Work out the finished part from the listing and answer in its coordinate system (mm). A direction names the side the tool comes from. Coordinates: 2 decimals unless noted, no trailing zeros. Order: outer loops, then holes, each group sorted by start corner. A loop starts at its lowest first (then second) coordinate and runs counter-clockwise, first axis right, second up. Notation, with made-up numbers: M 17.25,63.5 L 62.25,63.5 A18 cw 62.25,72.5 Z; hole C -40,-20.75 d11. An arc over 180 degrees is marked long. Use a Markdown table: item, result.
from build123d import *
from build123d.topology import SkipClean

# Parameters (mm, degrees)
BOSS_EXTRUDE1_START = 0.2
BOSS_EXTRUDE1_DEPTH = 5.6
BOSS_EXTRUDE2_DEPTH = 1.9
SKETCH5_R           = 1.65
BOSS_EXTRUDE3_DEPTH = 3
SKETCH6_W           = 5.7
SKETCH6_H           = 11.6
BOSS_EXTRUDE4_DEPTH = 0.6
BOSS_EXTRUDE5_START = -2
BOSS_EXTRUDE5_DEPTH = 5
SKETCH3_R           = 1.65
CUT_EXTRUDE1_DEPTH  = 50
BOSS_EXTRUDE6_START = -4
SKETCH10_R          = 4
SKETCH10_R_2        = 1.65
BOSS_EXTRUDE6_DEPTH = 4
CUT_EXTRUDE3_DEPTH  = 3
SKETCH13_R          = 1.65
CUT_EXTRUDE4_DEPTH  = 10
SKETCH14_R          = 3.25
CUT_EXTRUDE5_DEPTH  = 10
FILLET1_R           = 1


with BuildPart() as part:
    # Sketch2 → Boss-Extrude1 (new body)
    with BuildSketch(Plane.XZ.offset(22.088801204).offset(BOSS_EXTRUDE1_START)):
        with BuildLine():
            ThreePointArc((19.781498191, 14.5), (13.681498191, 8.4), (7.581498191, 14.5))
            Line((7.581498191, 14.5), (2.581498191, 14.5))
            Line((2.581498191, 14.5), (0.981498191, 14.5))
            Line((0.981498191, 14.5), (0.981498191, 0))
            Line((0.981498191, 0), (26.381498191, 0))
            Line((26.381498191, 0), (26.381498191, 14.5))
            Line((26.381498191, 14.5), (24.781498191, 14.5))
            Line((24.781498191, 14.5), (19.781498191, 14.5))
        make_face()
    extrude(amount=BOSS_EXTRUDE1_DEPTH)

    # Sketch4 → Boss-Extrude2 (add)
    with BuildSketch(Plane.XY):
        Polygon((5.781498191, -39.638801204), (5.781498191, -41.988801204), (31.081498191, -41.988801204), (31.081498191, -4.488801204), (-3.537114605, -4.488801204), (-3.537114605, -33.288801204), (2.722919547, -33.288801204), (5.781498191, -36.347379848), align=None)
    extrude(amount=BOSS_EXTRUDE2_DEPTH)

    # Sketch5 → Boss-Extrude3 (add)
    # profile 1 of 2: a face of its own
    with BuildSketch(Plane.XY.offset(1.9)):
        Polygon((-3.737114605, -9.588801204), (-10.195693249, -9.588801204), (-13.137114605, -12.53022256), (-13.137114605, -16.447379848), (-10.195693249, -19.388801204), (-3.737114605, -19.388801204), (-0.537114605, -19.388801204), (-0.537114605, -9.588801204), align=None)
        with Locations((-8.237114605, -14.488801204)):
            Circle(SKETCH5_R, mode=Mode.SUBTRACT)
    # profile 2 of 2: a face of its own
    with BuildSketch(Plane.XY.offset(1.9)):
        Polygon((5.781498191, -41.988801204), (-3.537114605, -41.988801204), (-3.537114605, -33.488801204), (-3.537114605, -32.143344659), (8.781498191, -32.143344659), (8.781498191, -41.988801204), align=None)
        with Locations((0.681498191, -37.638801204)):
            Circle(SKETCH5_R, mode=Mode.SUBTRACT)
    extrude(amount=BOSS_EXTRUDE3_DEPTH)

    # Sketch6 → Boss-Extrude4 (add)
    with BuildSketch(Plane.XY.offset(1.9)):
        with Locations((28.231498191, -22.988801204)):
            Rectangle(SKETCH6_W, SKETCH6_H)
    extrude(amount=BOSS_EXTRUDE4_DEPTH)

    # Sketch9 → Boss-Extrude5 (add)
    with BuildSketch(Plane(origin=(26.381498191, 0, 0), x_dir=(0, 0, -1), z_dir=(1, 0, 0)).offset(BOSS_EXTRUDE5_START)):
        Polygon((-1.9, -38.988801204), (-4.9, -38.988801204), (-14.5, -27.888801204), (-14.5, -22.288801204), (-4.9, -9.488801204), (-1.9, -9.488801204), align=None)
    boss_extrude5 = extrude(amount=BOSS_EXTRUDE5_DEPTH)

    # Sketch3 → Cut-Extrude1 (cut)
    with BuildSketch(Plane.XY.offset(14.5)):
        with Locations((22.781498191, -25.088801204)):
            Circle(SKETCH3_R)
    cut_extrude1 = extrude(amount=-CUT_EXTRUDE1_DEPTH, mode=Mode.SUBTRACT)

    # Sketch10 → Boss-Extrude6 (add)
    with BuildSketch(Plane(origin=(0, 0, 0), x_dir=(-1, 0, 0), z_dir=(0, 0, -1)).offset(BOSS_EXTRUDE6_START)):
        with Locations((-22.781498191, -25.088801204)):
            Circle(SKETCH10_R)
        with Locations(Location((-22.781498191, -25.088801204, 0), (0, 0, 180))):
            Circle(SKETCH10_R_2, mode=Mode.SUBTRACT)
    boss_extrude6 = extrude(amount=BOSS_EXTRUDE6_DEPTH)

    # Sketch11 → Cut-Extrude3 (cut)
    with BuildSketch(Plane(origin=(0, 0, 0), x_dir=(-1, 0, 0), z_dir=(0, 0, -1))):
        Polygon((-22.781498191, -21.913374723), (-25.531498191, -23.501087964), (-25.531498191, -26.676514444), (-22.781498191, -28.264227685), (-20.031498191, -26.676514444), (-20.031498191, -23.501087964), align=None)
    cut_extrude3 = extrude(amount=-CUT_EXTRUDE3_DEPTH, mode=Mode.SUBTRACT)

    # Mirror1: Boss-Extrude5, Cut-Extrude1, Boss-Extrude6, Cut-Extrude3 across plane
    add(boss_extrude5.mirror(Plane(origin=(13.681498191, 0, 0), x_dir=(0, 0, 1), z_dir=(1, 0, 0))))
    add(cut_extrude1.mirror(Plane(origin=(13.681498191, 0, 0), x_dir=(0, 0, 1), z_dir=(1, 0, 0))), mode=Mode.SUBTRACT)
    add(boss_extrude6.mirror(Plane(origin=(13.681498191, 0, 0), x_dir=(0, 0, 1), z_dir=(1, 0, 0))))
    add(cut_extrude3.mirror(Plane(origin=(13.681498191, 0, 0), x_dir=(0, 0, 1), z_dir=(1, 0, 0))), mode=Mode.SUBTRACT)

    # Sketch13 → Cut-Extrude4 (cut)
    with SkipClean():  # the faces are left unmerged after this step: merging them gives an invalid solid
        with BuildSketch(Plane(origin=(0, 0, 1.9), x_dir=(-1, 0, 0), z_dir=(0, 0, -1))):
            with Locations(Location((-0.681498191, -37.638801204, 0), (0, 0, 305.096801228))):
                Circle(SKETCH13_R)
        extrude(amount=-CUT_EXTRUDE4_DEPTH, mode=Mode.SUBTRACT)

    # Sketch14 → Cut-Extrude5 (cut)
    with SkipClean():  # the faces are left unmerged after this step: merging them gives an invalid solid
        with BuildSketch(Plane.XY.offset(4.9)):
            with Locations((0.681498191, -37.638801204)):
                Circle(SKETCH14_R)
        extrude(amount=CUT_EXTRUDE5_DEPTH, mode=Mode.SUBTRACT)

    # Fillet1
    fillet1_edges = [part.edges().sort_by_distance(p)[0] for p in [
        (2.981498191, -35.342608703, 6.476731892),
        (-2.018501809, -35.829795952, 6.266056325),
    ]]
    fillet(fillet1_edges, radius=FILLET1_R)


solid = part.part
(1) Straight lines are drawn through the part: L1, parallel to X at y = -13, z = 2.5; L2, parallel to X at y = -28, z = 1; L3, parallel to X at y = -21, z = 11.5. For each, find the intervals that lie inside material, in ascending order.
Conclusion:
| item | result |
|---|---|
| L1 | -13.14 to -8.95, -7.53 to 2.98, 24.38 to 29.38 |
| L2 | -3.54 to 4.12, 5.04 to 22.32, 23.24 to 31.08 |
| L3 | -2.02 to 2.98, 24.38 to 29.38 |
(2) Given P1, Ø1.5, axis at y = -11, z = 5, coming from the -X side; P2, Ø0.6, axis at y = -40.5, z = 1.5, coming from the -X side; P3, Ø4, axis at y = -14.5, z = 9.5, coming from the -X side; P4, Ø2, axis at x = -7.5, y = -22, coming from the +Z side, each flat-ended and moving along its own axis, determine where each tip first touches the part or whether it passes through.
Conclusion:
| item | result |
|---|---|
| P1 | x = -12.35 |
| P2 | x = 5.78 |
| P3 | x = -2.02 |
| P4 | through |
(3) Which of the six approach directions +Z, -Z, +X, -X, +Y, -Y give full straight-line access (tool end or side, diameter ignored) to faces 3 (the flat face through (24.176, -27.459, 1.479)), 4 (the flat face through (5, -22, 4)), 5 (the flat face through (-6, -9.589, 3)), 6 (the flat face through (8.781, -37, 3))?
Conclusion:
| item | result |
|---|---|
| face 3 | -Z |
| face 4 | +Z, +Y |
| face 5 | +Z, -X, +Y |
| face 6 | +Z, -Y |
(4) A cutting plane is placed at C-C (y = -14). Determine the outline of the cut face in (x, z), then the cut area to 3 significant figures.
Conclusion:
| item | result |
|---|---|
| outline | M -13.14,1.9 L -9.81,1.9 L -9.81,4.9 L -13.14,4.9 Z; M -6.66,1.9 L -3.54,1.9 L -3.54,0 L 31.08,0 L 31.08,1.9 L 29.38,1.9 L 29.38,8.28 L 24.38,8.28 L 24.38,1.9 L 2.98,1.9 L 2.98,8.28 L -2.02,8.28 L -2.02,4.9 L -6.66,4.9 Z |
| area | 154 mm2 |
(5) A cutting plane is placed at A-A (z = 13.5). Determine the outline of the cut face in (x, y).
Conclusion:
| item | result |
|---|---|
| outline | M -2.02,-29.05 L 2.98,-29.05 L 2.98,-27.89 L 7.66,-27.89 L 7.66,-22.29 L 2.98,-22.29 L 2.98,-20.96 L -2.02,-20.96 Z; M 19.7,-27.89 L 24.38,-27.89 L 24.38,-29.05 L 29.38,-29.05 L 29.38,-20.96 L 24.38,-20.96 L 24.38,-22.29 L 19.7,-22.29 Z; hole C 4.58,-25.09 d3.3; hole C 22.78,-25.09 d3.3 |
(6) Determine the mould class of faces 1 (the flat face through (30, -23, 2.5)), 2 (the flat face through (3.226, -22.696, 1.479)) for opening direction X: pulls with the +X half, pulls with the -X half, needs draft (parallel to the pull), parting line crosses it, or undercut.
Conclusion:
| item | result |
|---|---|
| face 1 | needs draft |
| face 2 | undercut |
(7) A cutting plane is placed at D-D (z = 7). Determine the outline of the cut face in (x, y), then the cut area to 3 significant figures.
Conclusion:
| item | result |
|---|---|
| outline | M -2.02,-33.74 A1 ccw -0.62,-34.66 A3.25 cw 1.68,-34.54 A1 ccw 2.98,-33.59 L 2.98,-27.89 L 24.38,-27.89 L 24.38,-36.56 L 29.38,-36.56 L 29.38,-12.29 L 24.38,-12.29 L 24.38,-22.29 L 2.98,-22.29 L 2.98,-12.29 L -2.02,-12.29 Z; hole C 4.58,-25.09 d3.3; hole C 22.78,-25.09 d3.3 |
| area | 335 mm2 |
(8) A cutting plane is placed at B-B (x = 23.5). Determine the outline of the cut face in (y, z).
Conclusion:
| item | result |
|---|---|
| outline | M -41.99,0 L -27.85,0 L -27.85,3 L -26.57,3 L -26.57,14.5 L -27.89,14.5 L -27.89,4 L -29.02,4 L -29.02,1.9 L -41.99,1.9 Z; M -23.6,3 L -22.33,3 L -22.33,0 L -4.49,0 L -4.49,1.9 L -21.15,1.9 L -21.15,4 L -22.29,4 L -22.29,14.5 L -23.6,14.5 Z |
